from build123d import *

# Parameters (mm, degrees)
CROQUIS1_R              = 3
SALIENTE_EXTRUIR1_DEPTH = 5
CORTAR_EXTRUIR1_START   = -5
CORTAR_EXTRUIR1_DEPTH   = 5
CORTAR_EXTRUIR2_DEPTH   = 10


# Read off the part's stored shape, not the designer's step: Cortar-Extruir1
with BuildPart() as part:
    # Croquis1 → Saliente-Extruir1 (new body)
    with BuildSketch(Plane(origin=(0, 0, 0), x_dir=(1, 0, 0), z_dir=(0, 1, 0))):
        with BuildLine():
            Line((-6, 7.413947971), (-6, 3.413947971))
            Line((-6, 3.413947971), (-3.653075314, 3.413947971))
            ThreePointArc((-3.653075314, 3.413947971), (0, -5), (3.653075314, 3.413947971))
            Line((3.653075314, 3.413947971), (6, 3.413947971))
            Line((6, 3.413947971), (6, 7.413947971))
            ThreePointArc((6, 7.413947971), (0, 5), (-6, 7.413947971))
        make_face()
        with Locations(Location((0, 0, 0), (0, 0, 270))):
            Circle(CROQUIS1_R, mode=Mode.SUBTRACT)
    extrude(amount=SALIENTE_EXTRUIR1_DEPTH)

    # Cortar-Extruir1 outline → Cortar-Extruir1 (cut)
    with BuildSketch(Plane(origin=(0, 5, 0), x_dir=(1, 0, 0), z_dir=(0, 1, 0)).offset(CORTAR_EXTRUIR1_START)):
        with BuildLine():
            Line((-2.974891432, -0.387325401), (-2.5, -4.330127019))
            ThreePointArc((-2.5, -4.330127019), (0, -5), (2.5, -4.330127019))
            Line((2.5, -4.330127019), (2.974891432, -0.387325401))
            ThreePointArc((2.974891432, -0.387325401), (0, -3), (-2.974891432, -0.387325401))
        make_face()
    extrude(amount=CORTAR_EXTRUIR1_DEPTH, mode=Mode.SUBTRACT)

    # Croquis3 → Cortar-Extruir2 (cut)
    with BuildSketch(Plane(origin=(0, 5, 0), x_dir=(1, 0, 0), z_dir=(0, 1, 0))):
        Polygon((3.653075314, 3.413947971), (6, 5.413947971), (6, 3.413947971), align=None)
        Polygon((-3.653075314, 3.413947971), (-6, 5.413947971), (-6, 3.413947971), align=None)
    extrude(amount=-CORTAR_EXTRUIR2_DEPTH, mode=Mode.SUBTRACT)


solid = part.part
Can you work these out from the model? Positions are in its coordinate system, mm. A direction names the side the tool comes from. Coordinates: 2 decimals unless noted, no trailing zeros. Write each loop counter-clockwise with the first axis right and the second up, starting at its lowest first coordinate (ties: lowest second). Pieces come first, ordered by that corner, then holes. Notation, with made-up numbers: (-23, 10.5) -> (33, 10.5) arc R23 ccw to (33, 40.5) -> close; hole circle Ø4 at (43, -32.75). An arc over 180 degrees is marked (long way). Write item = value, one per line.
(1) If I drill on probe 1 along X at (y, z) = (3.05, 0); probe 2 along Z at (x, y) = (4, 2.7); probe 3 along X at (y, z) = (0.45, -6.5), over which ranges is the centre line in solid material (lowest first)?
Verdict:
probe_1 = -5 to -3, 3 to 5
probe_2 = -5.98 to -3.71, -3 to 3
probe_3 = -6 to -4.87, 4.87 to 6
(2) On a 3-axis mill with a long thin cutter (end or side, diameter ignored), from which of +Z, -Z, +X, -X, +Y, -Y can I reach the whole of each face in a straight line? I mean faces 1 (the face through (4.81, 2.54, -4.4)), 2 (the face through (-4.954, 2.465, 0.674)), 3 (the face through (2.734, 2.465, 2.386)). Say none if no direction works.
Verdict:
face_1 = +X, +Y, -Y
face_2 = -X, +Y, -Y
face_3 = +Y, -Y
(3) Imagine slicing it at A-A (z = 0). Please give me the cut outline in (x, y), and give its area (3 significant figures).
Verdict:
outline = (-5, 0) -> (-3, 0) -> (-3, 5) -> (-5, 5) -> close; (3, 0) -> (5, 0) -> (5, 5) -> (3, 5) -> close
area = 20.0 mm^2
(4) Thinking about a two-plate mould opening in X: for faces 4 (the face through (6, 2, -6)), 5 (the face through (0, 2, -3)), 6 (the face through (0, 2, -5)), 7 (the face through (-4.81, 2.54, -4.4)), which applies, +X half, -X half, draft (parallel to the pull), parting line (faces both ways), or undercut?
Verdict:
face_4 = +X half
face_5 = undercut
face_6 = undercut
face_7 = -X half
(5) Imagine slicing it at D-D (z = -1.25). Please give me the cut outline in (x, y), and give its area (3 significant figures).
Verdict:
outline = (-4.84, 0) -> (-2.73, 0) -> (-2.73, 5) -> (-4.84, 5) -> close; (2.73, 0) -> (4.84, 0) -> (4.84, 5) -> (2.73, 5) -> close
area = 21.1 mm^2
(6) Imagine slicing it at B-B (y = 0.3). Please give me the cut outline in (x, z), and give its area (3 significant figures).
Verdict:
outline = (-6, -7.41) arc R8.66 cw to (6, -7.41) -> (6, -5.41) -> (3.65, -3.41) arc R5 ccw to (2.5, 4.33) -> (2.97, 0.39) arc R3 cw (long way) to (-2.97, 0.39) -> (-2.5, 4.33) arc R5 ccw to (-3.65, -3.41) -> (-6, -5.41) -> close
area = 53.6 mm^2
(7) For pin 1 (1.5 mm diameter, centred on x = -1.5, y = 1.5, fed in from -Z); pin 2 (1.5 mm diameter, centred on y = 1.5, z = 1, fed in from -X); pin 3 (1 mm diameter, centred on x = -4.5, y = 1.5, fed in from -Z), each with a flat end and sliding along its axis, tell me the tip position at first contact or that it passes through.
Verdict:
pin_1 = -5.3
pin_2 = -4.99
pin_3 = -6.59
(8) Imagine slicing it at C-C (x = 0). Please give me the cut outline in (y, z).
Verdict:
outline = (0, -5) -> (5, -5) -> (5, -3) -> (0, -3) -> close
